Geometry check sheet. Reference: the model listing, model coordinates, mm. A direction names the side the tool comes from. Coordinates: 2 decimals unless noted, no trailing zeros. Loops run counter-clockwise (first coordinate to the right, second up) from the corner with the lowest first, then second, coordinate; pieces in that order, holes last.
Autodesk Fusion 360 part; units mm, degrees
sketch "スケッチ1" plane through (0, 0, 0) normal (0, 1, 0) x (1, 0, 0)
  line L0 (0, 0) -> (74, 0)
  line L1 (74, 0) -> (74, -44)
  line L2 (74, -44) -> (0, -44)
  line L3 (0, -44) -> (0, 0)
  dimension "d1" = 74
  dimension "d2" = 44
extrude "押し出し1" add sketch "スケッチ1" along normal blind 2
sketch "スケッチ2" plane through (0, 0, 0) normal (0, -1, 0) x (1, 0, 0)
  line L0 (74, 44) -> (0, 44)
  line L1 (0, 44) -> (0, 0)
  line L2 (0, 0) -> (74, 0)
  line L3 (74, 0) -> (74, 44)
  line L4 (0, 44) -> (7, 44)
  line L5 (7, 44) -> (7, 42)
  line L6 (7, 42) -> (0, 42)
  line L7 (0, 42) -> (0, 44)
  line L8 (16, 42) -> (24, 42)
  line L9 (24, 42) -> (24, 44)
  line L10 (24, 44) -> (16, 44)
  line L11 (16, 44) -> (16, 42)
  line L12 (41, 44) -> (33, 44)
  line L13 (33, 42) -> (41, 42)
  line L14 (41, 42) -> (41, 44)
  line L15 (33, 44) -> (33, 42)
  line L16 (58, 44) -> (50, 44)
  line L17 (50, 42) -> (58, 42)
  line L18 (58, 42) -> (58, 44)
  line L19 (50, 44) -> (50, 42)
  line L20 (67, 42) -> (74, 42)
  line L21 (74, 42) -> (74, 44)
  line L22 (74, 44) -> (67, 44)
  line L23 (67, 44) -> (67, 42)
  line L24 (50, 2) -> (50, 0)
  line L25 (67, 2) -> (67, 0)
  line L26 (16, 0) -> (24, 0)
  line L27 (50, 0) -> (58, 0)
  line L28 (0, 2) -> (7, 2)
  line L29 (67, 0) -> (74, 0)
  line L30 (58, 0) -> (58, 2)
  line L31 (24, 2) -> (16, 2)
  line L32 (33, 2) -> (33, 0)
  line L33 (58, 2) -> (50, 2)
  line L34 (33, 0) -> (41, 0)
  line L35 (0, 0) -> (0, 2)
  line L36 (24, 0) -> (24, 2)
  line L37 (74, 2) -> (67, 2)
  line L38 (7, 2) -> (7, 0)
  line L39 (41, 0) -> (41, 2)
  line L40 (16, 2) -> (16, 0)
  line L41 (74, 0) -> (74, 2)
  line L42 (7, 0) -> (0, 0)
  line L43 (41, 2) -> (33, 2)
  dimension "d5" = 7
  dimension "d6" = 2
  dimension "d7" = 2
  dimension "d8" = 8
  dimension "d9" = 9
  dimension "d12" = 17
  dimension "d13" = 0
  dimension "d14" = 7
  dimension "d15" = 2
  dimension "d16" = 9
extrude "押し出し2" cut sketch "スケッチ2" against normal blind 2 contours L0 L3 L20 L21 L22 L23 | L0 L16 L17 L18 L19 | L2 L3 L25 L29 L37 L41 | L0 L12 L13 L14 L15 | L2 L24 L27 L30 L33 | L0 L8 L9 L10 L11 | L2 L32 L34 L39 L43 | L0 L1 L4 L5 L6 L7 | L2 L26 L31 L36 L40 | L1 L2 L28 L35 L38 L42
sketch "スケッチ3" plane through (0, 0, 0) normal (0, -1, 0) x (1, 0, 0)
  line L0 (33, 42) -> (33, 44)
  line L1 (33, 44) -> (24, 44)
  line L2 (24, 44) -> (24, 42)
  line L3 (24, 42) -> (16, 42)
  line L4 (16, 42) -> (16, 44)
  line L5 (16, 44) -> (7, 44)
  line L6 (7, 44) -> (7, 42)
  line L7 (7, 42) -> (0, 42)
  line L8 (0, 42) -> (0, 2)
  line L9 (0, 2) -> (7, 2)
  line L10 (7, 2) -> (7, 0)
  line L11 (7, 0) -> (16, 0)
  line L12 (16, 0) -> (16, 2)
  line L13 (16, 2) -> (24, 2)
  line L14 (24, 2) -> (24, 0)
  line L15 (24, 0) -> (33, 0)
  line L16 (33, 0) -> (33, 2)
  line L17 (33, 2) -> (41, 2)
  line L18 (41, 2) -> (41, 0)
  line L19 (41, 0) -> (50, 0)
  line L20 (50, 0) -> (50, 2)
  line L21 (50, 2) -> (58, 2)
  line L22 (58, 2) -> (58, 0)
  line L23 (58, 0) -> (67, 0)
  line L24 (67, 0) -> (67, 2)
  line L25 (67, 2) -> (74, 2)
  line L26 (74, 2) -> (74, 42)
  line L27 (74, 42) -> (67, 42)
  line L28 (67, 42) -> (67, 44)
  line L29 (67, 44) -> (58, 44)
  line L30 (58, 44) -> (58, 42)
  line L31 (58, 42) -> (50, 42)
  line L32 (50, 42) -> (50, 44)
  line L33 (50, 44) -> (41, 44)
  line L34 (41, 44) -> (41, 42)
  line L35 (41, 42) -> (33, 42)
  line L36 (2, 37) -> (0, 37)
  line L37 (0, 37) -> (0, 31)
  line L38 (0, 31) -> (2, 31)
  line L39 (2, 31) -> (2, 37)
  line L40 (0, 19) -> (2, 19)
  line L41 (0, 25) -> (0, 19)
  line L42 (2, 25) -> (0, 25)
  line L43 (2, 19) -> (2, 25)
  line L44 (0, 7) -> (2, 7)
  line L45 (0, 13) -> (0, 7)
  line L46 (2, 13) -> (0, 13)
  line L47 (2, 7) -> (2, 13)
  line L48 (72, 31) -> (74, 31)
  line L49 (74, 37) -> (72, 37)
  line L50 (74, 25) -> (72, 25)
  line L51 (72, 37) -> (72, 31)
  line L52 (72, 19) -> (74, 19)
  line L53 (72, 7) -> (74, 7)
  line L54 (74, 19) -> (74, 25)
  line L55 (72, 25) -> (72, 19)
  line L56 (74, 7) -> (74, 13)
  line L57 (74, 31) -> (74, 37)
  line L58 (72, 13) -> (72, 7)
  line L59 (74, 13) -> (72, 13)
  dimension "d23" = 7
  dimension "d24" = 6
  dimension "d25" = 2
  dimension "d28" = 0
  dimension "d29" = -12
  dimension "d30" = 7
  dimension "d33" = 72
  dimension "d34" = 0
extrude "押し出し3" cut sketch "スケッチ3" against normal blind 2 contours L8 L36 L37 L38 L39 | L26 L48 L49 L51 L57 | L8 L40 L41 L42 L43 | L26 L50 L52 L54 L55 | L8 L44 L45 L46 L47 | L26 L53 L56 L58 L59
sketch "スケッチ4" plane through (0, 0, 0) normal (0, -1, 0) x (1, 0, 0)
  line L0 (2, 31) -> (0, 31)
  line L1 (0, 31) -> (0, 25)
  line L2 (0, 25) -> (2, 25)
  line L3 (2, 25) -> (2, 19)
  line L4 (2, 19) -> (0, 19)
  line L5 (0, 19) -> (0, 13)
  line L6 (0, 13) -> (2, 13)
  line L7 (2, 13) -> (2, 7)
  line L8 (2, 7) -> (0, 7)
  line L9 (0, 7) -> (0, 2)
  line L10 (0, 2) -> (7, 2)
  line L11 (7, 2) -> (7, 0)
  line L12 (7, 0) -> (16, 0)
  line L13 (16, 0) -> (16, 2)
  line L14 (16, 2) -> (24, 2)
  line L15 (24, 2) -> (24, 0)
  line L16 (24, 0) -> (33, 0)
  line L17 (33, 0) -> (33, 2)
  line L18 (33, 2) -> (41, 2)
  line L19 (41, 2) -> (41, 0)
  line L20 (41, 0) -> (50, 0)
  line L21 (50, 0) -> (50, 2)
  line L22 (50, 2) -> (58, 2)
  line L23 (58, 2) -> (58, 0)
  line L24 (58, 0) -> (67, 0)
  line L25 (67, 0) -> (67, 2)
  line L26 (67, 2) -> (74, 2)
  line L27 (74, 2) -> (74, 7)
  line L28 (74, 7) -> (72, 7)
  line L29 (72, 7) -> (72, 13)
  line L30 (72, 13) -> (74, 13)
  line L31 (74, 13) -> (74, 19)
  line L32 (74, 19) -> (72, 19)
  line L33 (72, 19) -> (72, 25)
  line L34 (72, 25) -> (74, 25)
  line L35 (74, 25) -> (74, 31)
  line L36 (74, 31) -> (72, 31)
  line L37 (72, 31) -> (72, 37)
  line L38 (72, 37) -> (74, 37)
  line L39 (74, 37) -> (74, 42)
  line L40 (74, 42) -> (67, 42)
  line L41 (67, 42) -> (67, 44)
  line L42 (67, 44) -> (58, 44)
  line L43 (58, 44) -> (58, 42)
  line L44 (58, 42) -> (50, 42)
  line L45 (50, 42) -> (50, 44)
  line L46 (50, 44) -> (41, 44)
  line L47 (41, 44) -> (41, 42)
  line L48 (41, 42) -> (33, 42)
  line L49 (33, 42) -> (33, 44)
  line L50 (33, 44) -> (24, 44)
  line L51 (24, 44) -> (24, 42)
  line L52 (24, 42) -> (16, 42)
  line L53 (16, 42) -> (16, 44)
  line L54 (16, 44) -> (7, 44)
  line L55 (7, 44) -> (7, 42)
  line L56 (7, 42) -> (0, 42)
  line L57 (0, 42) -> (0, 37)
  line L58 (0, 37) -> (2, 37)
  line L59 (2, 37) -> (2, 31)
  line L60 (36, 15) -> (38, 15)
  line L61 (38, 15) -> (38, 25)
  line L62 (38, 25) -> (36, 25)
  line L63 (36, 25) -> (36, 15)
  line L64 (33, 15) -> (31, 15)
  line L65 (31, 15) -> (31, 25)
  line L66 (31, 25) -> (33, 25)
  line L67 (33, 25) -> (33, 15)
  line L68 (28, 15) -> (26, 15)
  line L69 (26, 15) -> (26, 25)
  line L70 (26, 25) -> (28, 25)
  line L71 (28, 25) -> (28, 15)
  line L72 (41, 15) -> (43, 15)
  line L73 (43, 15) -> (43, 25)
  line L74 (43, 25) -> (41, 25)
  line L75 (41, 25) -> (41, 15)
  line L76 (46, 15) -> (48, 15)
  line L77 (48, 15) -> (48, 25)
  line L78 (48, 25) -> (46, 25)
  line L79 (46, 25) -> (46, 15)
  line L80 (23, 15) -> (21, 15)
  line L81 (21, 15) -> (21, 25)
  line L82 (21, 25) -> (23, 25)
  line L83 (23, 25) -> (23, 15)
  line L84 (51, 15) -> (53, 15)
  line L85 (53, 15) -> (53, 25)
  line L86 (53, 25) -> (51, 25)
  line L87 (51, 25) -> (51, 15)
extrude "押し出し4" cut sketch "スケッチ4" against normal blind 2 contours L60 L61 L62 L63 | L64 L65 L66 L67 | L68 L69 L70 L71 | L72 L73 L74 L75 | L76 L77 L78 L79 | L80 L81 L82 L83 | L84 L85 L86 L87
sketch "スケッチ5" plane through (0, 0, 0) normal (0, -1, 0) x (1, 0, 0)
  line L0 (31, 15) -> (31, 25)
  line L1 (31, 25) -> (33, 25)
  line L2 (33, 25) -> (33, 15)
  line L3 (33, 15) -> (31, 15)
  line L4 (38, 15) -> (36, 15)
  line L5 (36, 15) -> (36, 25)
  line L6 (36, 25) -> (38, 25)
  line L7 (38, 25) -> (38, 15)
  line L8 (26, 15) -> (26, 25)
  line L9 (26, 25) -> (28, 25)
  line L10 (28, 25) -> (28, 15)
  line L11 (28, 15) -> (26, 15)
  line L12 (21, 15) -> (21, 25)
  line L13 (21, 25) -> (23, 25)
  line L14 (23, 25) -> (23, 15)
  line L15 (23, 15) -> (21, 15)
  line L16 (48, 15) -> (46, 15)
  line L17 (46, 15) -> (46, 25)
  line L18 (46, 25) -> (48, 25)
  line L19 (48, 25) -> (48, 15)
  line L20 (43, 15) -> (41, 15)
  line L21 (41, 15) -> (41, 25)
  line L22 (41, 25) -> (43, 25)
  line L23 (43, 25) -> (43, 15)
  line L24 (53, 15) -> (51, 15)
  line L25 (51, 15) -> (51, 25)
  line L26 (51, 25) -> (53, 25)
  line L27 (53, 25) -> (53, 15)
  line L28 (2, 31) -> (0, 31)
  line L29 (0, 31) -> (0, 25)
  line L30 (0, 25) -> (2, 25)
  line L31 (2, 25) -> (2, 19)
  line L32 (2, 19) -> (0, 19)
  line L33 (0, 19) -> (0, 13)
  line L34 (0, 13) -> (2, 13)
  line L35 (2, 13) -> (2, 7)
  line L36 (2, 7) -> (0, 7)
  line L37 (0, 7) -> (0, 2)
  line L38 (0, 2) -> (7, 2)
  line L39 (7, 2) -> (7, 0)
  line L40 (7, 0) -> (16, 0)
  line L41 (16, 0) -> (16, 2)
  line L42 (16, 2) -> (24, 2)
  line L43 (24, 2) -> (24, 0)
  line L44 (24, 0) -> (33, 0)
  line L45 (33, 0) -> (33, 2)
  line L46 (33, 2) -> (41, 2)
  line L47 (41, 2) -> (41, 0)
  line L48 (41, 0) -> (50, 0)
  line L49 (50, 0) -> (50, 2)
  line L50 (50, 2) -> (58, 2)
  line L51 (58, 2) -> (58, 0)
  line L52 (58, 0) -> (67, 0)
  line L53 (67, 0) -> (67, 2)
  line L54 (67, 2) -> (74, 2)
  line L55 (74, 2) -> (74, 7)
  line L56 (74, 7) -> (72, 7)
  line L57 (72, 7) -> (72, 13)
  line L58 (72, 13) -> (74, 13)
  line L59 (74, 13) -> (74, 19)
  line L60 (74, 19) -> (72, 19)
  line L61 (72, 19) -> (72, 25)
  line L62 (72, 25) -> (74, 25)
  line L63 (74, 25) -> (74, 31)
  line L64 (74, 31) -> (72, 31)
  line L65 (72, 31) -> (72, 37)
  line L66 (72, 37) -> (74, 37)
  line L67 (74, 37) -> (74, 42)
  line L68 (74, 42) -> (67, 42)
  line L69 (67, 42) -> (67, 44)
  line L70 (67, 44) -> (58, 44)
  line L71 (58, 44) -> (58, 42)
  line L72 (58, 42) -> (50, 42)
  line L73 (50, 42) -> (50, 44)
  line L74 (50, 44) -> (41, 44)
  line L75 (41, 44) -> (41, 42)
  line L76 (41, 42) -> (33, 42)
  line L77 (33, 42) -> (33, 44)
  line L78 (33, 44) -> (24, 44)
  line L79 (24, 44) -> (24, 42)
  line L80 (24, 42) -> (16, 42)
  line L81 (16, 42) -> (16, 44)
  line L82 (16, 44) -> (7, 44)
  line L83 (7, 44) -> (7, 42)
  line L84 (7, 42) -> (0, 42)
  line L85 (0, 42) -> (0, 37)
  line L86 (0, 37) -> (2, 37)
  line L87 (2, 37) -> (2, 31)
(1) Sectioned sample at A-A on z = 22. State how many separate pieces and enclosed holes the cut face has, and give its area (3 significant figures).
Findings:
separate pieces: 8
enclosed holes: 0
area: 112 mm2
(2) Gauge pin test, flat ends, axial feed: pin 1 Ø0.6 at (y, z) = (1.5, 20.5) entering from -X; pin 2 Ø0.6 at (y, z) = (1.5, 0.5) entering from -X; pin 3 Ø1 at (x, y) = (2.5, 1) entering from +Z. Record the tip position at first contact, or that the pin passes through.
Findings:
pin 1: stops at x = 2
pin 2: stops at x = 7
pin 3: stops at z = 42
(3) Draft check along Z on faces 4 (the flat face through (37, 1, 15)), 5 (the flat face through (37, 1, 2)), 6 (the flat face through (29, 1, 44)). Enter one of: +Z half, -Z half, draft (parallel to the pull), parting line (faces both ways), or undercut.
Findings:
face 4: undercut
face 5: -Z half
face 6: +Z half
(4) Sectioned sample at D-D on x = 18.5. Record the cut outline in (y, z), and give its area (3 significant figures).
Findings:
outline: (0, 2) - (2, 2) - (2, 42) - (0, 42) - close
area: 80.0 mm2
(5) Access from +Z, -Z, +X, -X, +Y, -Y to the whole of each face (thin tool, end or side, straight path). Record for faces 1 (the flat face through (22, 1, 15)), 2 (the flat face through (1, 1, 25)), 3 (the flat face through (50, 1, 43)).
Findings:
face 1: +Y, -Y
face 2: -X, +Y, -Y
face 3: +Z, +Y, -Y
(6) Scan lines: L1, parallel to Z at x = 47, y = 1.75; L2, parallel to Z at x = 6, y = 0.4; L3, parallel to X at y = 1.1, z = 8.5. Record each from-to range of solid material in increasing order.
Findings:
L1: z = 0 to 15, 25 to 44
L2: z = 2 to 42
L3: x = 2 to 72
